Input: part model. Units: mm. Frame: model coordinates. Face numbers are marked on the shaded views. A direction names the side the tool comes from. Give positions to 0.01 mm unless a question says otherwise; leave off trailing zeros. Loops run counter-clockwise (first coordinate to the right, second up) from the corner with the lowest first, then second, coordinate; pieces in that order, holes last. Notation, with made-up numbers: (-33.75, 34.5) - (11.25, 34.5) arc R27 ccw to (11.25, 72.5) - close; hole circle Ø7 at (29.5, -23.5). An arc over 180 degrees is marked (long way). Answer as a JSON object with one key per item and string values.
from build123d import *

# Parameters (mm, degrees)
SKETCH1_R           = 3.175
BOSS_EXTRUDE1_DEPTH = 7.62
SKETCH2_R           = 8.128
CUT_EXTRUDE1_DEPTH  = 5.08
SKETCH3_W           = 6.858
SKETCH3_H           = 6.858
CUT_EXTRUDE2_DEPTH  = 8.62
CHAMFER1_SIZE       = 1.27


with BuildPart() as part:
    # Sketch1 → Boss-Extrude1 (new body)
    with BuildSketch(Plane(origin=(0, 0, 0), x_dir=(1, 0, 0), z_dir=(0, 1, 0))):
        with BuildLine():
            ThreePointArc((-4.399409051, 24.642333042), (0, 27.182333042), (4.399409051, 24.642333042))
            Line((4.399409051, 24.642333042), (23.540590949, -8.511166521))
            ThreePointArc((23.540590949, -8.511166521), (23.540590949, -13.591166521), (19.141181898, -16.131166521))
            Line((19.141181898, -16.131166521), (-19.141181898, -16.131166521))
            ThreePointArc((-19.141181898, -16.131166521), (-23.540590949, -13.591166521), (-23.540590949, -8.511166521))
            Line((-23.540590949, -8.511166521), (-4.399409051, 24.642333042))
        make_face()
        Circle(SKETCH1_R, mode=Mode.SUBTRACT)
        with BuildLine():
            ThreePointArc((17.673352263, -12.403419212), (20.275630657, -11.706140818), (19.578352263, -9.103862424))
            Line((19.578352263, -9.103862424), (17.378647737, -7.833862424))
            ThreePointArc((17.378647737, -7.833862424), (14.776369343, -8.531140818), (15.473647737, -11.133419212))
            Line((15.473647737, -11.133419212), (17.673352263, -12.403419212))
        make_face(mode=Mode.SUBTRACT)
        with BuildLine():
            ThreePointArc((-15.473647737, -11.133419212), (-14.776369343, -8.531140818), (-17.378647737, -7.833862424))
            Line((-17.378647737, -7.833862424), (-19.578352263, -9.103862424))
            ThreePointArc((-19.578352263, -9.103862424), (-20.275630657, -11.706140818), (-17.673352263, -12.403419212))
            Line((-17.673352263, -12.403419212), (-15.473647737, -11.133419212))
        make_face(mode=Mode.SUBTRACT)
        with BuildLine():
            ThreePointArc((1.905, 21.507281636), (0, 23.412281636), (-1.905, 21.507281636))
            Line((-1.905, 21.507281636), (-1.905, 18.967281636))
            ThreePointArc((-1.905, 18.967281636), (0, 17.062281636), (1.905, 18.967281636))
            Line((1.905, 18.967281636), (1.905, 21.507281636))
        make_face(mode=Mode.SUBTRACT)
    extrude(amount=BOSS_EXTRUDE1_DEPTH)

    # Sketch2 → Cut-Extrude1 (cut)
    with BuildSketch(Plane.XZ):
        Circle(SKETCH2_R)
    extrude(amount=-CUT_EXTRUDE1_DEPTH, mode=Mode.SUBTRACT)

    # Sketch3 → Cut-Extrude2 (cut, through all)
    with BuildSketch(Plane(origin=(0, 0, 0), x_dir=(-1, 0, 0), z_dir=(0, -1, 0))):
        Rectangle(SKETCH3_W, SKETCH3_H)
    extrude(amount=-CUT_EXTRUDE2_DEPTH, mode=Mode.SUBTRACT)

    # Chamfer1
    chamfer1_edges = [part.edges().sort_by_distance(p)[0] for p in [
        (-8.128, 0, 0),
    ]]
    chamfer(chamfer1_edges, length=CHAMFER1_SIZE)


solid = part.part
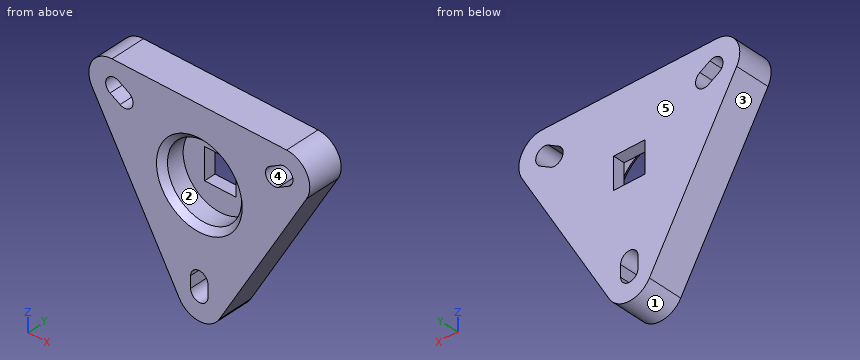
Item 1: Cut plane B-B (x = 0). Return loops of the section in (y, z).
Geometry check:
{"outline": "(0, -27.18) - (7.62, -27.18) - (7.62, -23.41) - (0, -23.41) - close; (0, -17.06) - (7.62, -17.06) - (7.62, -3.43) - (5.08, -3.43) - (5.08, -8.13) - (1.27, -8.13) - (0, -9.4) - close; (0, 9.4) - (1.27, 8.13) - (5.08, 8.13) - (5.08, 3.43) - (7.62, 3.43) - (7.62, 16.13) - (0, 16.13) - close"}
Item 2: Cut plane A-A (y = 2). Return loops of the section in (x, z) (3 decimals), then the cut area to 3 significant figures.
Geometry check:
{"outline": "(-23.541, 8.511) - (-4.399, -24.642) arc R5.08 ccw to (4.399, -24.642) - (23.541, 8.511) arc R5.08 ccw to (19.141, 16.131) - (-19.141, 16.131) arc R5.08 ccw to start; hole (-19.578, 9.104) - (-17.379, 7.834) arc R1.905 ccw to (-15.474, 11.133) - (-17.673, 12.403) arc R1.905 ccw to start; hole circle Ø16.256 at (0, 0); hole (-1.905, -21.507) arc R1.905 ccw to (1.905, -21.507) - (1.905, -18.967) arc R1.905 ccw to (-1.905, -18.967) - close; hole (15.474, 11.133) arc R1.905 ccw to (17.379, 7.834) - (19.578, 9.104) arc R1.905 ccw to (17.673, 12.403) - close", "area": "1,030 mm2"}
Item 3: Access query for the marked faces 1 and 2. Directions: +Z, -Z, +X, -X, +Y, -Y. A direction counts if a zero-diameter tool reaches every point of the face in a straight line with its end or side. Return the directions, or none.
Geometry check:
{"face 1": "-Z, +Y, -Y", "face 2": "-Y"}
Item 4: Contact query for flat-ended pins moving along their axis: P1, Ø0.8, axis at y = 7, z = -1.5, coming from the +X side; P2, Ø13, axis at x = -2, z = 0.5, coming from the -Y side; P3, Ø1.3, axis at y = 7, z = 0.5, coming from the -X side; P4, Ø18.5, axis at x = 0, z = 0, coming from the +Y side. Output: stop coordinate, or through.
Geometry check:
{"P1": "stops at x = 17.99", "P2": "stops at y = 0.84", "P3": "stops at x = -19.29", "P4": "stops at y = 7.62"}
Item 5: Mould query, pull axis Z, two halves, no side actions, for the marked faces 3, 4 and 5. Classes: released by +Z, released by -Z, zero draft, split by the parting line, or undercut.
Geometry check:
{"face 3": "released by -Z", "face 4": "undercut", "face 5": "zero draft"}
Item 6: Material intervals for line 1 (Z direction, x = 0, y = 2.2); line 2 (X direction, y = 6.25, z = 9.5); line 3 (Z direction, x = 20, y = 4), sorted ascending. Write a range as [from, to].
Geometry check:
{"line 1": "z = [-27.18, -23.41], [-17.06, -8.13], [8.13, 16.13]", "line 2": "x = [-23.98, -20.06], [-14.52, 14.52], [20.06, 23.98]", "line 3": "z = [2.38, 9.43], [12.07, 16.06]"}
Item 7: Cut plane C-C (z = 0). Return loops of the section in (x, y), then the cut area to 3 significant figures.
Geometry check:
{"outline": "(-18.63, 0) - (-9.4, 0) - (-8.13, 1.27) - (-8.13, 5.08) - (-3.43, 5.08) - (-3.43, 7.62) - (-18.63, 7.62) - close; (3.43, 5.08) - (8.13, 5.08) - (8.13, 1.27) - (9.4, 0) - (18.63, 0) - (18.63, 7.62) - (3.43, 7.62) - close", "area": "182 mm2"}
Item 8: Cut plane D-D (y = 6.5). Return loops of the section in (x, z) (3 decimals).
Geometry check:
{"outline": "(-23.541, 8.511) - (-4.399, -24.642) arc R5.08 ccw to (4.399, -24.642) - (23.541, 8.511) arc R5.08 ccw to (19.141, 16.131) - (-19.141, 16.131) arc R5.08 ccw to start; hole (-19.578, 9.104) - (-17.379, 7.834) arc R1.905 ccw to (-15.474, 11.133) - (-17.673, 12.403) arc R1.905 ccw to start; hole (-3.429, -3.429) - (3.429, -3.429) - (3.429, 3.429) - (-3.429, 3.429) - close; hole (-1.905, -21.507) arc R1.905 ccw to (1.905, -21.507) - (1.905, -18.967) arc R1.905 ccw to (-1.905, -18.967) - close; hole (15.474, 11.133) arc R1.905 ccw to (17.379, 7.834) - (19.578, 9.104) arc R1.905 ccw to (17.673, 12.403) - close"}
